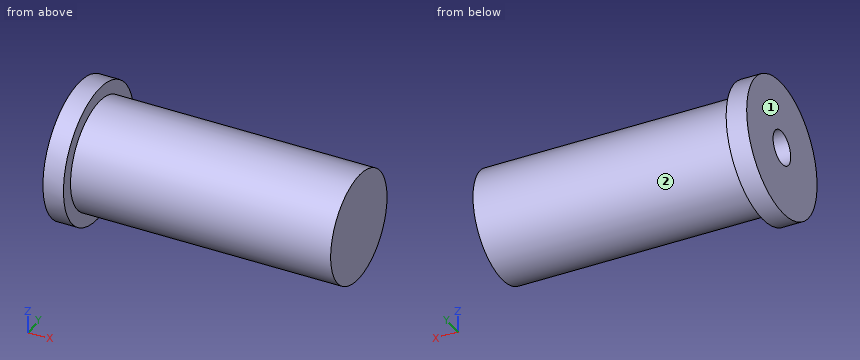
Autodesk Inventor part; units mm, degrees
ref_plane "YZ Plane" through (0, 0, 0) normal (1, 0, 0) x (0, 1, 0)
ref_plane "XZ Plane" through (0, 0, 0) normal (0, 1, 0) x (-1, 0, 0)
ref_plane "XY Plane" through (0, 0, 0) normal (0, 0, 1) x (1, 0, 0)
sketch "スケッチ1" plane through (0, 0, 0) normal (0, 0, 1) x (1, 0, 0)
  line L0 (0, 0) -> (0, 5)
  line L1 (0, 5) -> (1.5, 5)
  line L2 (1.5, 5) -> (1.5, 4)
  line L3 (1.5, 4) -> (20.5, 4)
  line L4 (20.5, 4) -> (20.5, 0)
  line L5 (20.5, 0) -> (0, 0)
  dimension "d0" = 5
  dimension "d1" = 1.5
  dimension "d2" = 4
  dimension "d3" = 20.5
revolve "回転1" add sketch "スケッチ1" angle 360 about axis through (20.5, 0, 0) along (-1, 0, 0)
sketch "スケッチ2" plane through (0, 0, 0) normal (-1, 0, 0) x (0, 0, 1)
  circle A0 centre (0, 0) radius 1.25
  dimension "d5" = 2.5
extrude "押し出し1" cut sketch "スケッチ2" against normal blind 15
properties part number "Circuit_MJ165H"
Part model, mm, in its own coordinate system. Face numbers are marked on the shaded views. A direction names the side the tool comes from. Give positions to 0.01 mm unless a question says otherwise; leave off trailing zeros. Loops run counter-clockwise (first coordinate to the right, second up) from the corner with the lowest first, then second, coordinate; pieces in that order, holes last. Notation, with made-up numbers: M -14,-35 L 5,-35 A11 ccw 5,-17 Z; hole C 27,6 d11. An arc over 180 degrees is marked long. Put each result on its own line as item: value. Start each with the question number.
1) Saw through at C-C (x = 2.5). List the corners of the cut face in (y, z).
2) Probe probe 1 along Y at (x, z) = (4.5, 0); probe 2 along X at (y, z) = (4, 1.5); probe 3 along Y at (x, z) = (3.5, 2.75). List the from-to ranges inside material, lowest first.
3) Saw through at A-A (y = 0). List the corners of the cut face in (x, z), then the cut area to 4 significant figures.
4) Saw through at D-D (x = 18.75). List the corners of the cut face in (y, z), then the cut area to 3 significant figures.
5) Flat gauge pins, fed straight in: pin 1 (3 mm diameter, centred on y = -0.5, z = -0.5, fed in from -X); pin 2 (2 mm diameter, centred on x = 6, y = -4, fed in from +Z); pin 3 (5 mm diameter, centred on x = 6.5, y = 1, fed in from -Z); pin 4 (1 mm diameter, centred on x = 6, y = 2, fed in from +Z). Where does each tip first touch, or does it go through?
6) 3-axis set-ups, long thin cutter, end or side, ignore diameter. For the marked faces 1 and 2: which of +Z, -Z, +X, -X, +Y, -Y reach the whole face in a straight line?
Numbers:
1. outline: C 0,0 d8; hole C 0,0 d2.5
2. probe 1: -4 to -1.25, 1.25 to 4
2. probe 2: 0 to 1.5
2. probe 3: -2.9 to 2.9
3. outline: M 0,-5 L 1.5,-5 L 1.5,-4 L 20.5,-4 L 20.5,4 L 1.5,4 L 1.5,5 L 0,5 L 0,1.25 L 15,1.25 L 15,-1.25 L 0,-1.25 Z
3. area: 129.5 mm^2
4. outline: C 0,0 d8
4. area: 50.3 mm^2
5. pin 1: x = 0
5. pin 2: z = 2.65
5. pin 3: z = -4
5. pin 4: z = 3.71
6. face 1: +Z, -Z, -X, +Y, -Y
6. face 2: +X
